Check sheet for the modelled part. Datum: model origin and axes. Units: mm. Round coordinates to 2 decimals unless told otherwise and drop trailing zeros. Loops run counter-clockwise (first coordinate to the right, second up) from the corner with the lowest first, then second, coordinate; pieces in that order, holes last. Notation, with made-up numbers: (63.25, -13.75) - (117.25, -13.75) arc R15 ccw to (117.25, -5.75) - close; hole circle Ø6 at (-6, 80). An arc over 180 degrees is marked (long way). Answer in a Markdown table with one row per item. Add a question column.
(1) Cross-section at A-A on y = 0. Enter the section's corners in (x, z), then the cut area to 3 significant figures.
(2) Thickness scan on line 1 along Y through (x, z) = (0, 2.9); line 2 along Y through (x, z) = (3.5, 1.95); line 3 along X through (y, z) = (-9, 3.4). Record the ranges inside material, lowest first.
(3) Cross-section at B-B on x = 0. Enter the section's corners in (y, z).
(4) Gauge pin test, flat end, axial feed: pin 1 (8 mm diameter, centred on x = 12.5, y = -17.5, fed in from -Z). Record the tip position at first contact, or that the pin passes through.
(5) Cross-section at C-C on z = 3.1. Enter the section's corners in (x, y).
Autodesk Inventor part; units mm, degrees
ref_plane "YZ Plane" through (0, 0, 0) normal (1, 0, 0) x (0, 1, 0)
ref_plane "XZ Plane" through (0, 0, 0) normal (0, 1, 0) x (-1, 0, 0)
ref_plane "XY Plane" through (0, 0, 0) normal (0, 0, 1) x (1, 0, 0)
sketch "Sketch1" plane through (0, 0, 0) normal (0, 0, 1) x (1, 0, 0)
  line L0 (-58.7375, -39.6875) -> (58.7375, -39.6875)
  line L1 (58.7375, -39.6875) -> (58.7375, 39.6875)
  line L2 (58.7375, 39.6875) -> (-58.7375, 39.6875)
  line L3 (-58.7375, 39.6875) -> (-58.7375, -39.6875)
  line L4 (-58.7375, -39.6875) -> (58.7375, 39.6875) construction
  line L5 (58.7375, -39.6875) -> (-58.7375, 39.6875) construction
  point P0 (0, 0)
  dimension "d0" = 117.475
  dimension "d1" = 79.375
extrude "Extrusion1" add sketch "Sketch1" along normal blind 4.7625
sketch "Sketch2" plane through (0, 0, 4.7625) normal (0, 0, 1) x (1, 0, 0)
  circle A0 centre (0, 0) radius 12.7
  dimension "d4" = 25.4
extrude "Extrusion2" cut sketch "Sketch2" against normal through all
properties part number "Back"
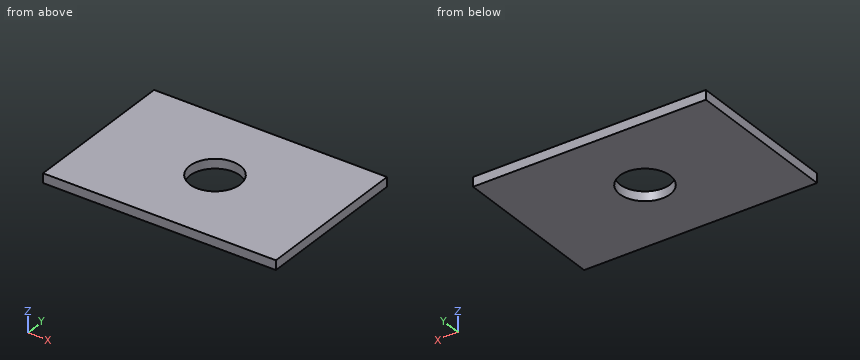
Answers:
| question | item | result |
|---|---|---|
| 1 | outline | (-58.74, 0) - (-12.7, 0) - (-12.7, 4.76) - (-58.74, 4.76) - close; (12.7, 0) - (58.74, 0) - (58.74, 4.76) - (12.7, 4.76) - close |
| 1 | area | 439 mm^2 |
| 2 | line 1 | y = -39.69 to -12.7, 12.7 to 39.69 |
| 2 | line 2 | y = -39.69 to -12.21, 12.21 to 39.69 |
| 2 | line 3 | x = -58.74 to -8.96, 8.96 to 58.74 |
| 3 | outline | (-39.69, 0) - (-12.7, 0) - (-12.7, 4.76) - (-39.69, 4.76) - close; (12.7, 0) - (39.69, 0) - (39.69, 4.76) - (12.7, 4.76) - close |
| 4 | pin 1 | stops at z = 0 |
| 5 | outline | (-58.74, -39.69) - (58.74, -39.69) - (58.74, 39.69) - (-58.74, 39.69) - close; hole circle Ø25.4 at (0, 0) |
